from build123d import *

# Parameters (mm, degrees)
F0_R     = 6.5
F1_DEPTH = 29
F2_R     = 5.75
F3_DEPTH = 15
F4_R     = 4
F5_DEPTH = 5
F6_R     = 5.75
F7_DEPTH = 15
F8_R     = 4
F9_DEPTH = 5
F10_R    = 1


with BuildPart() as f1:
    # F0 (on Front) → F1 (new body)
    with BuildSketch(Plane.XZ):
        Circle(F0_R)
    extrude(amount=F1_DEPTH)

    # F2 (on Front) → F3 (join)
    with BuildSketch(Plane.XZ):
        Circle(F2_R)
    extrude(amount=-F3_DEPTH)



with BuildPart() as f5:
    # F4 (on face) → F5 (new body)
    with BuildSketch(Plane.XZ.offset(44)):
        Circle(F4_R)
    extrude(amount=F5_DEPTH)


with BuildPart() as f1_1:
    add(f1.part)

    add(f5.part)  # F7 merges F5
    # F6 (on face) → F7 (join)
    with BuildSketch(Plane.XZ.offset(29)):
        Circle(F6_R)
    extrude(amount=F7_DEPTH)

    # F8 (on face) → F9 (join)
    with BuildSketch(Plane(origin=(0, 15, 0), x_dir=(-1, 0, 0), z_dir=(0, 1, 0))):
        Circle(F8_R)
    extrude(amount=F9_DEPTH)

    # F10
    f10_edges = [f1_1.edges().sort_by_distance(p)[0] for p in [
        (4, 20, 0),
        (-4, -49, 0),
    ]]
    fillet(f10_edges, radius=F10_R)


solid = f1_1.part
The model under review builds one solid part; all positions refer to its coordinate system, in mm. A direction names the side the tool comes from. Round coordinates to 2 decimals unless told otherwise and drop trailing zeros. Write each loop counter-clockwise with the first axis right and the second up, starting at its lowest first coordinate (ties: lowest second). Pieces come first, ordered by that corner, then holes. Notation, with made-up numbers: (47.25, -13) -> (101.25, -13) arc R10 cw to (101.25, 4) -> close; hole circle Ø8 at (73, 19). An arc over 180 degrees is marked (long way). Answer as a JSON object with one key per item and string values.
1. To check wall thickness, follow line 1 along Z through (x, y) = (0, -39.5); line 2 along Y through (x, z) = (2.5, 5.5); line 3 along Y through (x, z) = (3.25, -3). State the ranges of each line that lie inside material, in increasing order.
Results found:
{"line 1": "z = -5.75 to 5.75", "line 2": "y = -29 to 0", "line 3": "y = -44 to 15"}
2. We need section C-C on y = 5.5. State the section outline as (x, z) points, and give its area (3 significant figures).
Results found:
{"outline": "circle Ø11.5 at (0, 0)", "area": "104 mm^2"}
3. We need section D-D on x = -4.75. State the section outline as (y, z) points.
Results found:
{"outline": "(-44, -3.24) -> (-29, -3.24) -> (-29, -4.44) -> (0, -4.44) -> (0, -3.24) -> (15, -3.24) -> (15, 3.24) -> (0, 3.24) -> (0, 4.44) -> (-29, 4.44) -> (-29, 3.24) -> (-44, 3.24) -> close"}
4. We need section A-A on x = 0. State the section outline as (y, z) points, and give its area (3 significant figures).
Results found:
{"outline": "(-49, -3) arc R1 ccw to (-48, -4) -> (-44, -4) -> (-44, -5.75) -> (-29, -5.75) -> (-29, -6.5) -> (0, -6.5) -> (0, -5.75) -> (15, -5.75) -> (15, -4) -> (19, -4) arc R1 ccw to (20, -3) -> (20, 3) arc R1 ccw to (19, 4) -> (15, 4) -> (15, 5.75) -> (0, 5.75) -> (0, 6.5) -> (-29, 6.5) -> (-29, 5.75) -> (-44, 5.75) -> (-44, 4) -> (-48, 4) arc R1 ccw to (-49, 3) -> close", "area": "801 mm^2"}
5. Machinability: for faces 1 (the face through (2, -44, -4)), 2 (the face through (-5.158, -14.297, -3.955)), 3 (the face through (2, 15, -4)), which of the approach directions +Z, -Z, +X, -X, +Y, -Y give a long, thin tool a straight path to every point of the face, cutting with its end or side? Answer none if there is none.
Results found:
{"face 1": "-Y", "face 2": "+Y, -Y", "face 3": "+Y"}
6. We need section B-B on z = 0. State the section outline as (x, y) points, and give its area (3 significant figures).
Results found:
{"outline": "(-6.5, -29) -> (-5.75, -29) -> (-5.75, -44) -> (-4, -44) -> (-4, -48) arc R1 ccw to (-3, -49) -> (3, -49) arc R1 ccw to (4, -48) -> (4, -44) -> (5.75, -44) -> (5.75, -29) -> (6.5, -29) -> (6.5, 0) -> (5.75, 0) -> (5.75, 15) -> (4, 15) -> (4, 19) arc R1 ccw to (3, 20) -> (-3, 20) arc R1 ccw to (-4, 19) -> (-4, 15) -> (-5.75, 15) -> (-5.75, 0) -> (-6.5, 0) -> close", "area": "801 mm^2"}
7. Clearance check with flat-ended pins moving along their axes: pin 1 (1.5 mm diameter, centred on x = 5, y = -5.5, fed in from -Z); pin 2 (6 mm diameter, centred on y = -33.5, z = 0.5, fed in from +X); pin 3 (4 mm diameter, centred on x = 0, y = 2.5, fed in from -Z). State where each tip first meets the part, or that it passes through.
Results found:
{"pin 1": "stops at z = -4.92", "pin 2": "stops at x = 5.75", "pin 3": "stops at z = -5.75"}
